Design review of the part built by this model. Coordinates are the model's own, in mm. A direction names the side the tool comes from. Round coordinates to 2 decimals unless told otherwise and drop trailing zeros. Write each loop counter-clockwise with the first axis right and the second up, starting at its lowest first coordinate (ties: lowest second). Pieces come first, ordered by that corner, then holes. Notation, with made-up numbers: (58.5, -38.75) -> (84.5, -38.75) arc R29 cw to (84.5, -10.75) -> close; hole circle Ø4 at (60, -39.5). An arc over 180 degrees is marked (long way). Write item = value, one per line. Start each with the question number.
Item 1: Mouldability with a two-part tool opening along X and no side actions: class faces 1 (the cylindrical face through (23.846, 7.509, 3.574)), 2 (the flat face through (-8, 13, 7.25)), 3 (the cylindrical face through (23, 0, 4)) as released by +X, released by -X, zero draft, split by the parting line, or undercut.
Item 2: Add section A-A, the plane y = 0. State the section outline as (x, z) points, then the cut area to 3 significant figures.
Item 3: Add section C-C, the plane z = 6.5. State the section outline as (x, y) points.
Item 4: To check wall thickness, follow L1, parallel to X at y = 7, z = 6.25; L2, parallel to Y at x = 5.5, z = 6; L3, parallel to Y at x = 16, z = 3.75. State the ranges of each line that lie inside material, in increasing order.
Item 5: Machinability: for faces 4 (the flat face through (-9, 16, 2)), 5 (the flat face through (-6.84, 11.99, 4.59)), which of the approach directions +Z, -Z, +X, -X, +Y, -Y give a long, thin tool a straight path to every point of the face, cutting with its end or side? Answer none if there is none.
Item 6: For pin 1 Ø5.5 at (x, y) = (11.5, -13.5) entering from -Z; pin 2 Ø3 at (y, z) = (-13, 2) entering from -X, all flat-tipped, find the tip position at first contact; note any pin that passes through.
Item 7: Add section D-D, the plane x = -20. State the section outline as (y, z) points.
from build123d import *

# Parameters (mm, degrees)
SKETCH1_R             = 25
BOSS_EXTRUDE1_DEPTH   = 7.25
F_3_0MM_DOWEL_HOLE1_D = 3
CIRPATTERN1_COUNT     = 3
CUT_EXTRUDE7_DEPTH    = 8.25
CUT_EXTRUDE9_DEPTH    = 2


with BuildPart() as part:
    # Sketch1 → Boss-Extrude1 (new body)
    with BuildSketch(Plane.XY):
        Circle(SKETCH1_R)
    extrude(amount=BOSS_EXTRUDE1_DEPTH)

    # Ø3.0mm Dowel Hole1 (through all)
    with Locations(Plane(origin=(0, 0, 0), x_dir=(-1, 0, 0), z_dir=(0, 0, -1))):
        with Locations((-15.552844037, 14.110600354)):
            f_3_0mm_dowel_hole1 = Hole(F_3_0MM_DOWEL_HOLE1_D / 2)

    # CirPattern1: Ø3.0mm Dowel Hole1 ×3 about axis
    cirpattern1_axis = Axis((0, 0, 0), (0, 0, 1))
    for i in range(1, CIRPATTERN1_COUNT):
        add(f_3_0mm_dowel_hole1.rotate(cirpattern1_axis, i * 360 / CIRPATTERN1_COUNT), mode=Mode.SUBTRACT)

    # Sketch4 → Cut-Extrude7 (cut, through all)
    with BuildSketch(Plane(origin=(0, 0, 0), x_dir=(-1, 0, 0), z_dir=(0, 0, -1))):
        with BuildLine():
            Line((8.755064083, 21.268494373), (4.272899712, 13.463995507))
            Line((4.272899712, 13.463995507), (9.475898956, 10.475885926))
            Line((9.475898956, 10.475885926), (13.958063327, 18.280384792))
            ThreePointArc((13.958063327, 18.280384792), (18.328536057, 13.894774774), (21.370809866, 8.502263561))
            ThreePointArc((21.370809866, 8.502263561), (17.616017485, 5.650303353), (22.329156288, 5.514415606))
            ThreePointArc((22.329156288, 5.514415606), (17.034067279, -15.454467055), (-3.3222287, -22.758796024))
            ThreePointArc((-3.3222287, -22.758796024), (-3.9147025, -18.081070332), (-6.388954142, -22.094824393))
            ThreePointArc((-6.388954142, -22.094824393), (-10.232582573, -20.598404159), (-13.747128962, -18.439534845))
            Line((-13.747128962, -18.439534845), (-7.472625388, -11.987356538))
            Line((-7.472625388, -11.987356538), (-11.774077593, -7.804354156))
            Line((-11.774077593, -7.804354156), (-18.048581167, -14.256532463))
            ThreePointArc((-18.048581167, -14.256532463), (-23, 0), (-18.048581167, 14.256532463))
            ThreePointArc((-18.048581167, 14.256532463), (-13.701314985, 12.430766979), (-15.940202146, 16.580408787))
            ThreePointArc((-15.940202146, 16.580408787), (-4.289649037, 22.596435806), (8.755064083, 21.268494373))
        make_face()
    extrude(amount=-CUT_EXTRUDE7_DEPTH, mode=Mode.SUBTRACT)

    # Sketch9 → Cut-Extrude9 (cut)
    with BuildSketch(Plane(origin=(0, 0, 0), x_dir=(-1, 0, 0), z_dir=(0, 0, -1))):
        Polygon((-11.774077593, -7.804354156), (-18.048581167, -14.256532463), (-13.747128962, -18.439534845), (-7.472625388, -11.987356538), align=None)
        Polygon((4.272899712, 13.463995507), (8.755064083, 21.268494373), (13.958063327, 18.280384792), (9.475898956, 10.475885926), align=None)
    extrude(amount=-CUT_EXTRUDE9_DEPTH, mode=Mode.SUBTRACT)


solid = part.part
Result set:
q1.face_1 = split by the parting line
q1.face_2 = zero draft
q1.face_3 = undercut
q2.outline = (-25, 0) -> (-23, 0) -> (-23, 7.25) -> (-25, 7.25) -> close; (23, 0) -> (25, 0) -> (25, 7.25) -> (23, 7.25) -> close
q2.area = 29.0 mm²
q3.outline = circle Ø50 at (0, 0); hole (-22.33, 5.51) arc R23 ccw to (3.32, -22.76) arc R2.5 cw (long way) to (6.39, -22.09) arc R23 ccw to (13.75, -18.44) -> (7.47, -11.99) -> (11.77, -7.8) -> (18.05, -14.26) arc R23 ccw to (18.05, 14.26) arc R2.5 cw (long way) to (15.94, 16.58) arc R23 ccw to (-8.76, 21.27) -> (-4.27, 13.46) -> (-9.48, 10.48) -> (-13.96, 18.28) arc R23 ccw to (-21.37, 8.5) arc R2.5 cw (long way) to start; hole circle Ø3 at (-20, 6.41); hole circle Ø3 at (4.44, -20.52); hole circle Ø3 at (15.55, 14.11)
q4.L1 = -24 to -21.38, -18.62 to -17.57, 21.91 to 24
q4.L2 = -24.39 to -21.59, -19.46 to -18.26, 22.33 to 24.39
q4.L3 = -19.21 to -12.15, 11.65 to 12.68, 15.54 to 19.21
q5.face_4 = -Z
q5.face_5 = +Z, -Z
q6.pin_1 = 2
q6.pin_2 = -22.2
q7.outline = (-15, 0) -> (-11.36, 0) -> (-11.36, 7.25) -> (-15, 7.25) -> close; (3.91, 0) -> (4.91, 0) -> (4.91, 7.25) -> (3.91, 7.25) -> close; (7.91, 0) -> (8.91, 0) -> (8.91, 7.25) -> (7.91, 7.25) -> close; (11.36, 0) -> (15, 0) -> (15, 7.25) -> (11.36, 7.25) -> close
